Autodesk Inventor part; units mm, degrees
ref_plane "YZ Plane" through (0, 0, 0) normal (1, 0, 0) x (0, 1, 0)
ref_plane "XZ Plane" through (0, 0, 0) normal (0, 1, 0) x (-1, 0, 0)
ref_plane "XY Plane" through (0, 0, 0) normal (0, 0, 1) x (1, 0, 0)
sketch "スケッチ1" plane through (0, 0, 0) normal (0, 0, 1) x (1, 0, 0)
  circle A0 centre (0, 0) radius 1.5
  dimension "d0" = 3
extrude "押し出し1" add sketch "スケッチ1" along normal blind 8
chamfer "面取り1" distance 0.134 distance2 0.5 1 edges at (-1.5, 0, 8) measured on face at (0.3743, -0.3316, 8)
chamfer "面取り2" distance 0.134 distance2 0.5 1 edges at (-1.5, 0, 0) measured on face at (0.3743, -0.3316, 0)
properties part number "平行ピンΦ3.8" material "鋼、高強度、低合金"
The model under review builds one solid part; all positions refer to its coordinate system, in mm. Give positions to 0.01 mm unless a question says otherwise; leave off trailing zeros. Loops run counter-clockwise (first coordinate to the right, second up) from the corner with the lowest first, then second, coordinate; pieces in that order, holes last. Notation, with made-up numbers: (75.5, -3) -> (92.5, -3) arc R28 ccw to (92.5, 27) -> close; hole circle Ø8 at (-19, -3). An arc over 180 degrees is marked (long way). Write each question's results on one line, items separated by ' | '.
1) Insertion check: pin 1 Ø1 at (x, z) = (-1, 2.5) entering from -Y. The pin has a flat end and moves straight along its axis. Give the tip position at first contact, or say it passes through.
Conclusion:
pin 1: stops at y = -1.41
2) For line 1 along Y through (x, z) = (0.95, 3.25); line 2 along Y through (x, z) = (-0.35, 4.5); line 3 along X through (y, z) = (0.85, 6.75), list the stretches that pass through material, from the lowest coordinate up. Write a range as from..to.
Conclusion:
line 1: y = -1.16..1.16 | line 2: y = -1.46..1.46 | line 3: x = -1.24..1.24
3) Take a section at A-A, the plane z = 4.25. Give the boundary of the cut face in (x, y).
Conclusion:
outline: circle Ø3 at (0, 0)
